```python
from build123d import *

# Parameters (mm, degrees)
SKETCH1_W           = 8.8
SKETCH1_H           = 8.8
BOSS_EXTRUDE1_DEPTH = 5.5
SKETCH2_W           = 17.6
SKETCH2_H           = 8.8
BOSS_EXTRUDE2_DEPTH = 0.1
SKETCH3_R           = 2.617377511
BOSS_EXTRUDE3_DEPTH = 1


with BuildPart() as part:
    # Sketch1 → Boss-Extrude1 (new body)
    with BuildSketch(Plane.XY):
        Rectangle(SKETCH1_W, SKETCH1_H)
    extrude(amount=BOSS_EXTRUDE1_DEPTH)

    # Sketch2 → Boss-Extrude2 (add)
    with BuildSketch(Plane(origin=(0, 0, 0), x_dir=(-1, 0, 0), z_dir=(0, 0, -1))):
        with Locations((-4.4, 0)):
            Rectangle(SKETCH2_W, SKETCH2_H)
    extrude(amount=-BOSS_EXTRUDE2_DEPTH)

    # Sketch3 → Boss-Extrude3 (add)
    with BuildSketch(Plane.XY.offset(5.5)):
        Circle(SKETCH3_R)
    extrude(amount=BOSS_EXTRUDE3_DEPTH)


solid = part.part
```
Geometry: final body of the model. Coordinates: model frame, mm. A direction names the side the tool comes from. Round coordinates to 2 decimals unless told otherwise and drop trailing zeros. Loops run counter-clockwise (first coordinate to the right, second up) from the corner with the lowest first, then second, coordinate; pieces in that order, holes last. Notation, with made-up numbers: (72.5, 23) -> (79.5, 23) arc R21 ccw to (79.5, 51) -> close; hole circle Ø1 at (4.25, 50.5). An arc over 180 degrees is marked (long way). Write each question's results on one line, items separated by ' | '.
Item 1: Pin query (flat end, axial travel): pin 1 Ø2 at (y, z) = (2.5, 4) entering from +X. Return the tip coordinate at first contact, or that it passes through.
Answers below:
pin 1: stops at x = 4.4
Item 2: Line query: probe 1 along X at (y, z) = (-2.25, 5.25); probe 2 along X at (y, z) = (-1, 6.25); probe 3 along Y at (x, z) = (-2.25, 6). Output: solid intervals per line, ascending. Write a range as [from, to].
Answers below:
probe 1: x = [-4.4, 4.4] | probe 2: x = [-2.42, 2.42] | probe 3: y = [-1.34, 1.34]
Item 3: Cut plane C-C on z = 5.25. Return the cut outline in (x, y).
Answers below:
outline: (-4.4, -4.4) -> (4.4, -4.4) -> (4.4, 4.4) -> (-4.4, 4.4) -> close
Item 4: Set-up query: faces 1 (the face through (-2, -2, 5.5)), 2 (the face through (1, -4.4, 3)), 3 (the face through (4.4, 0, 3)). Return all of +Z, -Z, +X, -X, +Y, -Y with unobstructed straight access to the full face (end or side cutting, diameter ignored); none if empty.
Answers below:
face 1: +Z | face 2: +Z, -Z, +X, -X, -Y | face 3: +Z, +X, +Y, -Y
Item 5: Cut plane D-D on x = 4. Return the cut outline in (y, z).
Answers below:
outline: (-4.4, 0) -> (4.4, 0) -> (4.4, 5.5) -> (-4.4, 5.5) -> close
Item 6: Cut plane A-A on x = 0. Return the cut outline in (y, z), and give its area (3 significant figures).
Answers below:
outline: (-4.4, 0) -> (4.4, 0) -> (4.4, 5.5) -> (2.62, 5.5) -> (2.62, 6.5) -> (-2.62, 6.5) -> (-2.62, 5.5) -> (-4.4, 5.5) -> close | area: 53.6 mm²
Item 7: Cut plane B-B on y = 0. Return the cut outline in (x, z).
Answers below:
outline: (-4.4, 0) -> (13.2, 0) -> (13.2, 0.1) -> (4.4, 0.1) -> (4.4, 5.5) -> (2.62, 5.5) -> (2.62, 6.5) -> (-2.62, 6.5) -> (-2.62, 5.5) -> (-4.4, 5.5) -> close
